Geometry: see drawing. Coordinates: mm, zero at the bounding-box minimum. A direction names the side the tool comes from. Coordinates: 2 decimals unless noted, no trailing zeros. Loops run counter-clockwise (first coordinate to the right, second up) from the corner with the lowest first, then second, coordinate; pieces in that order, holes last.
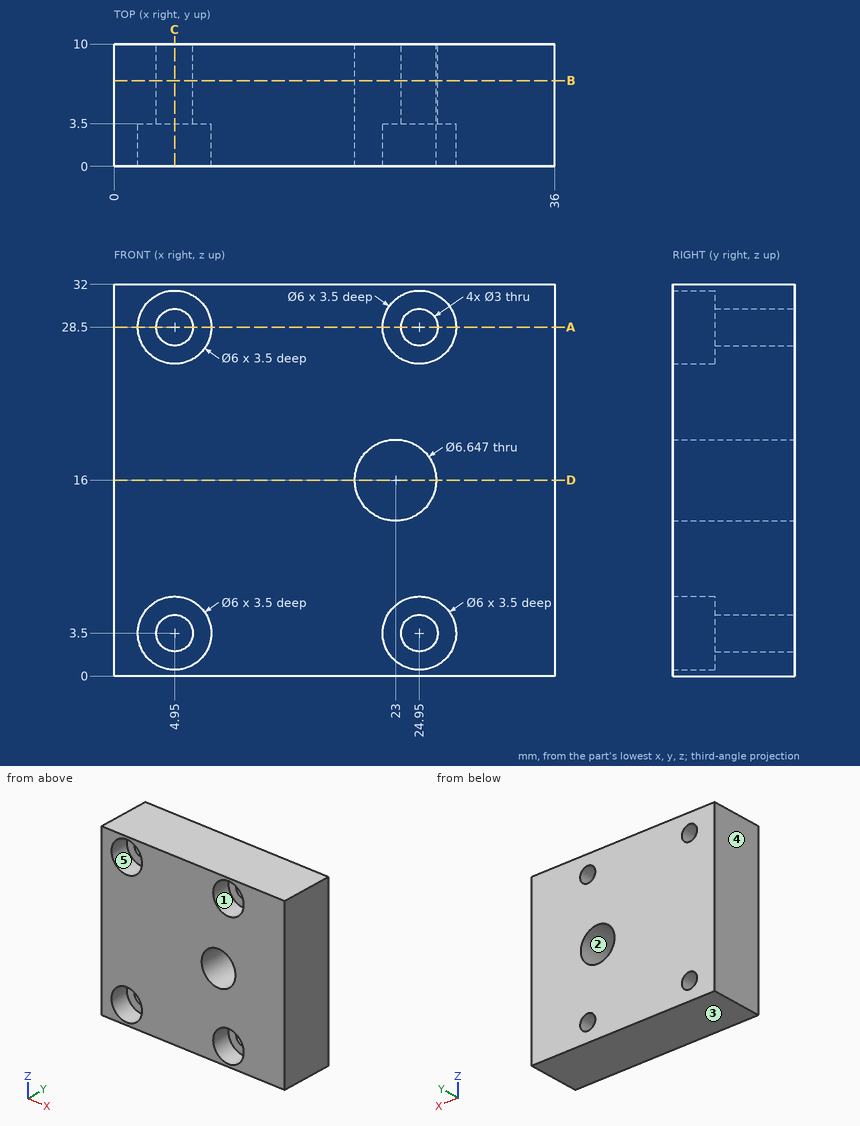
Item 1: Line query: L1, parallel to Z at x = 4.95, y = 6.5; L2, parallel to X at y = 8, z = 28.5; L3, parallel to Z at x = 24.95, y = 7.25. Output: solid intervals per line, ascending.
Result:
L1: z = 0 to 2, 5 to 27, 30 to 32
L2: x = 0 to 3.45, 6.45 to 23.45, 26.45 to 36
L3: z = 0 to 2, 5 to 13.31, 18.69 to 27, 30 to 32
Item 2: Section query B-B (y = 7). Output: boundary loops of the cut face in (x, z).
Result:
outline: (0, 0) - (36, 0) - (36, 32) - (0, 32) - close; hole circle Ø3 at (4.95, 3.5); hole circle Ø3 at (4.95, 28.5); hole circle Ø6.65 at (23, 16); hole circle Ø3 at (24.95, 3.5); hole circle Ø3 at (24.95, 28.5)
Item 3: Reachability of the marked faces 1 and 2 from +Z, -Z, +X, -X, +Y, -Y: full face, straight path, thin tool, end or side. Return the list, or none.
Result:
face 1: -Y
face 2: +Y, -Y
Item 4: Contact query for a flat-ended pin moving along its axis: P1, Ø3, axis at x = 24, z = 3.5, coming from the -Y side. Output: stop coordinate, or through.
Result:
P1: stops at y = 3.5
Item 5: Section query C-C (x = 4.95). Output: boundary loops of the cut face in (y, z).
Result:
outline: (0, 0) - (10, 0) - (10, 2) - (3.5, 2) - (3.5, 0.5) - (0, 0.5) - close; (0, 6.5) - (3.5, 6.5) - (3.5, 5) - (10, 5) - (10, 27) - (3.5, 27) - (3.5, 25.5) - (0, 25.5) - close; (0, 31.5) - (3.5, 31.5) - (3.5, 30) - (10, 30) - (10, 32) - (0, 32) - close
Item 6: Mould query, pull axis X, two halves, no side actions, for the marked faces 3, 4 and 5. Classes: +X half, -X half, draft (parallel to the pull), parting line (faces both ways), or undercut.
Result:
face 3: draft
face 4: -X half
face 5: undercut
Item 7: Section query A-A (z = 28.5). Output: boundary loops of the cut face in (x, y), then the cut area to 3 significant figures.
Result:
outline: (0, 0) - (1.95, 0) - (1.95, 3.5) - (3.45, 3.5) - (3.45, 10) - (0, 10) - close; (6.45, 3.5) - (7.95, 3.5) - (7.95, 0) - (21.95, 0) - (21.95, 3.5) - (23.45, 3.5) - (23.45, 10) - (6.45, 10) - close; (26.45, 3.5) - (27.95, 3.5) - (27.95, 0) - (36, 0) - (36, 10) - (26.45, 10) - close
area: 279 mm2
Item 8: Section query D-D (z = 16). Output: boundary loops of the cut face in (x, y), then the cut area to 3 significant figures.
Result:
outline: (0, 0) - (19.68, 0) - (19.68, 10) - (0, 10) - close; (26.32, 0) - (36, 0) - (36, 10) - (26.32, 10) - close
area: 294 mm2
